Read the model definition and answer for the solid it produces. Units are mm, in the model's axes. Face numbers are marked on the shaded views. A direction names the side the tool comes from. Coordinates: 2 decimals unless noted, no trailing zeros. Loops run counter-clockwise (first coordinate to the right, second up) from the corner with the lowest first, then second, coordinate; pieces in that order, holes last. Notation, with made-up numbers: M -14,26 L 6,26 A21 ccw 6,37 Z; hole C 78.5,-21 d2. An arc over 180 degrees is marked long. Put each result on its own line as item: value.
from build123d import *

# Parameters (mm, degrees)
SKETCH_1_W          = 10
SKETCH_1_H          = 10
SKETCH_1_W_2        = 8
SKETCH_1_H_2        = 8
EXTRUDE_1_DEPTH     = 28
SKETCH_4_R          = 2.1
CUT_EXTRUDE_3_DEPTH = 31.149626863
SKETCH_5_R          = 2.1
CUT_EXTRUDE_4_DEPTH = 31.149626863
SKETCH_6_R          = 4
CUT_EXTRUDE_5_DEPTH = 1


with BuildPart() as part:
    # ｽｹｯﾁ1 → 押し出し-薄板1 (new body)
    with BuildSketch(Plane(origin=(0, 0, 0), x_dir=(0, 0, -1), z_dir=(1, 0, 0))):
        Rectangle(SKETCH_1_W, SKETCH_1_H)
        Rectangle(SKETCH_1_W_2, SKETCH_1_H_2, mode=Mode.SUBTRACT)
    extrude(amount=EXTRUDE_1_DEPTH)

    # ｽｹｯﾁ4 → ｶｯﾄ - 押し出し3 (cut, through all)
    with BuildSketch(Plane.XY.offset(5)):
        with Locations((23, 0)):
            Circle(SKETCH_4_R)
        with Locations(Location((5, 0, 0), (0, 0, 90))):
            Circle(SKETCH_4_R)
    extrude(amount=-CUT_EXTRUDE_3_DEPTH, mode=Mode.SUBTRACT)

    # ｽｹｯﾁ5 → ｶｯﾄ - 押し出し4 (cut, through all)
    with BuildSketch(Plane(origin=(0, 5, 0), x_dir=(1, 0, 0), z_dir=(0, 1, 0))):
        with Locations(Location((15.5, 1, 0), (0, 0, 270))):
            Circle(SKETCH_5_R)
    extrude(amount=-CUT_EXTRUDE_4_DEPTH, mode=Mode.SUBTRACT)

    # ｽｹｯﾁ6 → ｶｯﾄ - 押し出し5 (cut)
    with BuildSketch(Plane(origin=(0, 0, -5), x_dir=(-1, 0, 0), z_dir=(0, 0, -1))):
        with Locations(Location((-5, 0, 0), (0, 0, 90))):
            Circle(SKETCH_6_R)
    extrude(amount=-CUT_EXTRUDE_5_DEPTH, mode=Mode.SUBTRACT)


solid = part.part
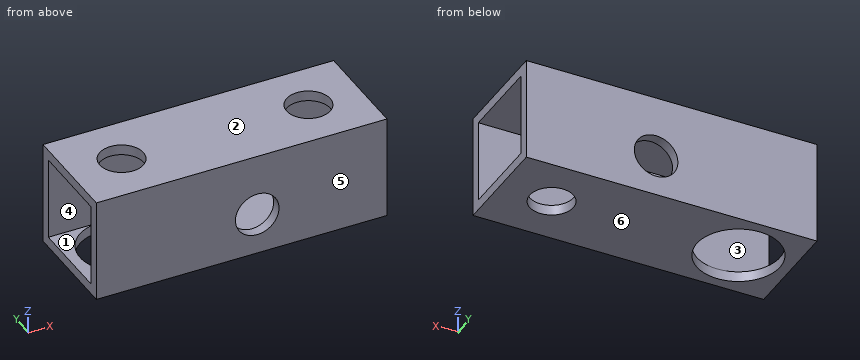
1) Find section A-A, the plane z = 2.75. Write down the section's boundary in (x, y).
Answer list:
outline: M 0,-5 L 28,-5 L 28,-4 L 0,-4 Z; M 0,4 L 28,4 L 28,5 L 0,5 Z
2) Find section D-D, the plane z = -0.5. Write down the section's boundary in (x, y), plus the area to 3 significant figures.
Answer list:
outline: M 0,-5 L 13.46,-5 L 13.46,-4 L 0,-4 Z; M 0,4 L 13.46,4 L 13.46,5 L 0,5 Z; M 17.54,-5 L 28,-5 L 28,-4 L 17.54,-4 Z; M 17.54,4 L 28,4 L 28,5 L 17.54,5 Z
area: 47.8 mm^2
3) Straight lines are drawn through the part: line 1 (Y direction, x = 1.5, z = -2.5); line 2 (X direction, y = 4.75, z = -1). For each, find the intervals that lie inside material, in ascending order. Write a range as [from, to].
Answer list:
line 1: y = [-5, -4], [4, 5]
line 2: x = [0, 13.4], [17.6, 28]
4) Determine the mould class of the marked faces 3, 4, 5 and 6 for opening direction Y: released by +Y, released by -Y, zero draft, split by the parting line, or undercut.
Answer list:
face 3: undercut
face 4: undercut
face 5: released by -Y
face 6: zero draft
5) Given pin 1 Ø6 at (y, z) = (0.5, 2.5) entering from -X; pin 2 Ø3.5 at (x, y) = (23, 0) entering from +Z, each flat-ended and moving along its own axis, determine where each tip first touches the part or whether it passes through.
Answer list:
pin 1: stops at x = 0
pin 2: passes through
6) Which of the six approach directions +Z, -Z, +X, -X, +Y, -Y give full straight-line access (tool end or side, diameter ignored) to the marked faces 1 and 2?
Answer list:
face 1: +X, -X
face 2: +Z, +X, -X, +Y, -Y
7) Find section C-C, the plane x = 19. Write down the section's boundary in (y, z), plus the area to 3 significant figures.
Answer list:
outline: M -5,-5 L 5,-5 L 5,5 L -5,5 Z; hole M -4,-4 L 4,-4 L 4,4 L -4,4 Z
area: 36.0 mm^2
8) Find section B-B, the plane y = 0. Write down the section's boundary in (x, z).
Answer list:
outline: M 0,-5 L 1,-5 L 1,-4 L 0,-4 Z; M 0,4 L 2.9,4 L 2.9,5 L 0,5 Z; M 7.1,4 L 20.9,4 L 20.9,5 L 7.1,5 Z; M 9,-5 L 20.9,-5 L 20.9,-4 L 9,-4 Z; M 25.1,-5 L 28,-5 L 28,-4 L 25.1,-4 Z; M 25.1,4 L 28,4 L 28,5 L 25.1,5 Z
